Work out the finished part from the listing and answer in its coordinate system (mm). Face numbers are marked on the shaded views. A direction names the side the tool comes from. Round coordinates to 2 decimals unless told otherwise and drop trailing zeros. Loops run counter-clockwise (first coordinate to the right, second up) from the corner with the lowest first, then second, coordinate; pieces in that order, holes last. Notation, with made-up numbers: (53, 68) - (88, 68) arc R11 ccw to (88, 80) - close; hole circle Ø8 at (16, 53). An arc over 180 degrees is marked (long way). Return JSON: item names as keys, results as strings.
from build123d import *

# Parameters (mm, degrees)
CROQUIS1_R              = 4
CROQUIS1_R_2            = 1.5
SALIENTE_EXTRUIR1_DEPTH = 8
CROQUIS2_W              = 23
CROQUIS2_H              = 8
CORTAR_EXTRUIR1_DEPTH   = 2.5
REDONDEO1_R             = 7
REDONDEO3_R             = 2


with BuildPart() as part:
    # Croquis1 → Saliente-Extruir1 (new body)
    # profile 1 of 2: a face of its own
    with BuildSketch(Plane.XY):
        Circle(CROQUIS1_R)
        Circle(CROQUIS1_R_2, mode=Mode.SUBTRACT)
    # profile 2 of 2: a face of its own
    with BuildSketch(Plane.XY):
        with BuildLine():
            ThreePointArc((4, 0), (2.828427125, -2.828427125), (0, -4))
            Line((0, -4), (37, -4))
            Line((37, -4), (37, 0))
            Line((37, 0), (4, 0))
        make_face()
    extrude(amount=SALIENTE_EXTRUIR1_DEPTH)

    # Croquis2 → Cortar-Extruir1 (cut)
    with BuildSketch(Plane(origin=(0, 0, 0), x_dir=(1, 0, 0), z_dir=(0, 1, 0))):
        with Locations((25.5, -4)):
            Rectangle(CROQUIS2_W, CROQUIS2_H)
    extrude(amount=-CORTAR_EXTRUIR1_DEPTH, mode=Mode.SUBTRACT)

    # Redondeo1
    redondeo1_edges = [part.edges().sort_by_distance(p)[0] for p in [
        (37, -3.25, 8),
    ]]
    fillet(redondeo1_edges, radius=REDONDEO1_R)

    # Redondeo3
    redondeo3_edges = [part.edges().sort_by_distance(p)[0] for p in [
        (37, -3.25, 0),
    ]]
    fillet(redondeo3_edges, radius=REDONDEO3_R)


solid = part.part
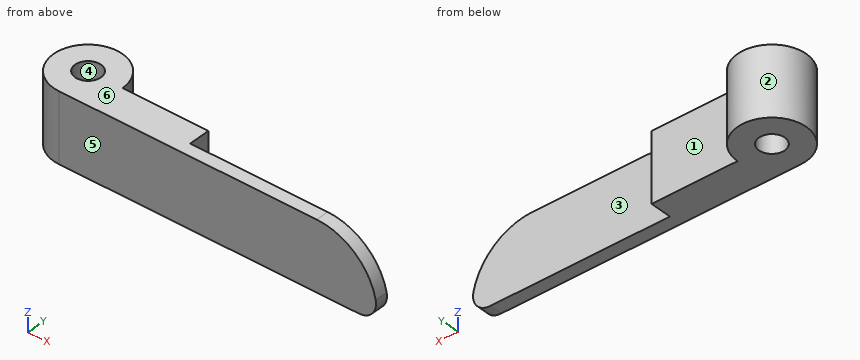
1) Determine the mould class of the marked faces 3, 4, 5 and 6 for opening direction Y: pulls with the +Y half, pulls with the -Y half, needs draft (parallel to the pull), parting line crosses it, or undercut.
Verdict:
{"face 3": "pulls with the +Y half", "face 4": "undercut", "face 5": "pulls with the -Y half", "face 6": "needs draft"}
2) Section B-B (z = 3.75) is taken. Give the vertices of the cut face in (x, y), and give its area (3 significant figures).
Verdict:
{"outline": "(0, -4) - (36.44, -4) - (36.44, -2.5) - (14, -2.5) - (14, 0) - (4, 0) arc R4 ccw (long way) to start; hole circle Ø3 at (0, 0)", "area": "120 mm2"}
3) A tool of negligible diameter and unlimited length cuts with its end or side. For the marked faces 1 and 2, from which of +Z, -Z, +X, -X, +Y, -Y can it reach the whole face along a straight path? Write none if from no direction.
Verdict:
{"face 1": "+Z, -Z, +X, +Y", "face 2": "+Z, -Z"}
4) Flat-ended cylindrical pins translate along their axes: pin 1 (3 mm diameter, centred on x = 32.5, y = -2.5, fed in from +Z); pin 2 (4 mm diameter, centred on x = 15, z = 7, fed in from +Y); pin 3 (1 mm diameter, centred on y = 3, z = 6.5, fed in from +X). Find the tip coordinate at first contact, or state that the pin passes through.
Verdict:
{"pin 1": "stops at z = 7.93", "pin 2": "stops at y = 0", "pin 3": "stops at x = 3.12"}
5) Section D-D (z = 7) is taken. Give the vertices of the cut face in (x, y).
Verdict:
{"outline": "(0, -4) - (33.61, -4) - (33.61, -2.5) - (14, -2.5) - (14, 0) - (4, 0) arc R4 ccw (long way) to start; hole circle Ø3 at (0, 0)"}
6) Section C-C (x = 18) is taken. Give the vertices of the cut face in (y, z), and give its area (3 significant figures).
Verdict:
{"outline": "(-4, 0) - (-2.5, 0) - (-2.5, 8) - (-4, 8) - close", "area": "12.0 mm2"}
7) Section A-A (y = -0.5) is taken. Give the vertices of the cut face in (x, z).
Verdict:
{"outline": "(-3.97, 0) - (-1.41, 0) - (-1.41, 8) - (-3.97, 8) - close; (1.41, 0) - (14, 0) - (14, 8) - (1.41, 8) - close"}
8) Find the intervals of material crossed by L1, parallel to Y at x = 18, z = 7; L2, parallel to X at y = 1, z = 5.25; L3, parallel to Y at x = 0.5, z = 3.5, in increasing order.
Verdict:
{"L1": "y = -4 to -2.5", "L2": "x = -3.87 to -1.12, 1.12 to 3.87", "L3": "y = -4 to -1.41, 1.41 to 3.97"}
